Design review of the part built by this model. Coordinates are the model's own, in mm. Face numbers are marked on the shaded views. A direction names the side the tool comes from. Round coordinates to 2 decimals unless told otherwise and drop trailing zeros. Loops run counter-clockwise (first coordinate to the right, second up) from the corner with the lowest first, then second, coordinate; pieces in that order, holes last. Notation, with made-up numbers: (37, 70) - (50, 70) arc R23 ccw to (50, 93) - close; hole circle Ø11 at (-23, 10). An arc over 180 degrees is marked (long way). Return JSON: item names as keys, results as strings. Group by question number.
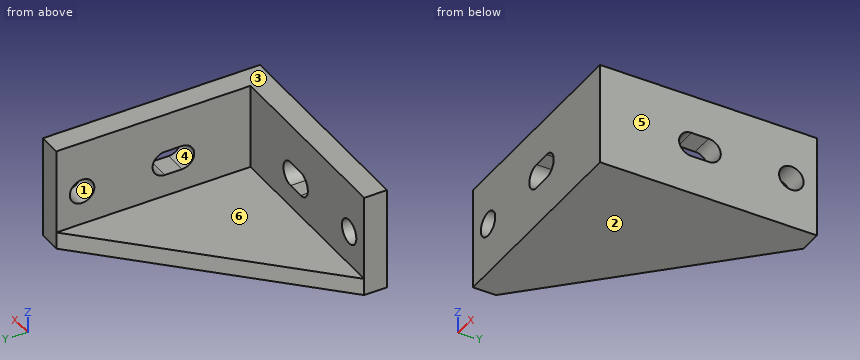
from build123d import *

# Parameters (mm, degrees)
EXTRUDE_1_DEPTH     = 9
EXTRUDE_2_DEPTH     = 3
SKETCH_4_R          = 2.15
CUT_EXTRUDE_1_DEPTH = 52.778373864


with BuildPart() as part:
    # 草图1 → 凸台-拉伸1 (new, symmetric)
    with BuildSketch(Plane.XY):
        Polygon((-38, 0), (0, 0), (0, 38), (-4, 38), (-4, 4), (-38, 4), align=None)
    extrude(amount=EXTRUDE_1_DEPTH, both=True)

    # 草图3 → 凸台-拉伸2 (add)
    with BuildSketch(Plane(origin=(0, 0, -9), x_dir=(-1, 0, 0), z_dir=(0, 0, -1))):
        Polygon((38, 4), (4, 38), (4, 4), align=None)
    extrude(amount=-EXTRUDE_2_DEPTH)

    # 草图4 → 切除-拉伸1 (cut, through all)
    with BuildSketch(Plane(origin=(0, 4, 0), x_dir=(1, 0, 0), z_dir=(0, 1, 0))):
        with Locations(Location((-33.5, 0, 0), (0, 0, 270))):
            Circle(SKETCH_4_R)
        with BuildLine():
            Line((-16, -2.15), (-19, -2.15))
            ThreePointArc((-19, -2.15), (-21.15, 0), (-19, 2.15))
            Line((-19, 2.15), (-16, 2.15))
            ThreePointArc((-16, 2.15), (-13.85, 0), (-16, -2.15))
        make_face()
    cut_extrude_1 = extrude(amount=-CUT_EXTRUDE_1_DEPTH, mode=Mode.SUBTRACT)

    # 镜向1: 切除-拉伸1 across plane
    add(cut_extrude_1.mirror(Plane(origin=(0, 0, 0), x_dir=(0, 0, 1), z_dir=(-0.7071067811865477, -0.7071067811865475, 0))), mode=Mode.SUBTRACT)


solid = part.part
Q1. Add section A-A, the plane z = 0. State the section outline as (x, y) points, plus the area to 3 significant figures.
Q2. For line 1 (X direction, y = 0.8, z = 0); line 2 (Y direction, x = -2.45, z = 0); line 3 (Z direction, x = -18, y = 3), list the stretches that pass through material, from the lowest coordinate up.
Q3. Draft analysis for pull direction Z (two halves, no side actions). For the marked faces 1, 2 and 3, state which applies: pulls with the +Z half, pulls with the -Z half, needs draft (parallel to the pull), parting line crosses it, or undercut.
Q4. Insertion check: pin 1 Ø1 at (x, z) = (-20.5, 5) entering from +Y; pin 2 Ø10 at (y, z) = (24, 7) entering from -X; pin 3 Ø17 at (x, y) = (-18.5, 13) entering from +Z. Each pin has a flat end and moves straight along its axis. Give the tip position at first contact, or say it passes through.
Q5. Add section D-D, the plane x = -8. State the section outline as (y, z) points.
Q6. Add section B-B, the plane y = 33.5. State the section outline as (x, z) points, plus the area to 3 significant figures.
Q7. Add section C-C, the plane x = -20.5. State the section outline as (y, z) points, plus the area to 3 significant figures.
Q8. Tool access review of the marked faces 4, 5 and 6: name each direction out of +Z, -Z, +X, -X, +Y, -Y from which nothing blocks a thin tool from reaching the whole face with its end or side.
Evaluation:
{
 "1": {"outline": "(-38, 0) - (-35.65, 0) - (-35.65, 4) - (-38, 4) - close; (-31.35, 0) - (-21.15, 0) - (-21.15, 4) - (-31.35, 4) - close; (-13.85, 0) - (0, 0) - (0, 13.85) - (-4, 13.85) - (-4, 4) - (-13.85, 4) - close; (-4, 21.15) - (0, 21.15) - (0, 31.35) - (-4, 31.35) - close; (-4, 35.65) - (0, 35.65) - (0, 38) - (-4, 38) - close", "area": "195 mm²"},
 "2": {"line 1": "-38 to -35.65, -31.35 to -21.15, -13.85 to 0", "line 2": "0 to 13.85, 21.15 to 31.35, 35.65 to 38", "line 3": "-9 to -2.15, 2.15 to 9"},
 "3": {"face 1": "undercut", "face 2": "pulls with the -Z half", "face 3": "pulls with the +Z half"},
 "4": {"pin 1": "y = 4", "pin 2": "x = -4", "pin 3": "z = -6"},
 "5": {"outline": "(0, -9) - (34, -9) - (34, -6) - (4, -6) - (4, 9) - (0, 9) - close"},
 "6": {"outline": "(-8.5, -9) - (0, -9) - (0, -2.15) - (-4, -2.15) - (-4, -6) - (-8.5, -6) - close; (-4, 2.15) - (0, 2.15) - (0, 9) - (-4, 9) - close", "area": "68.3 mm²"},
 "7": {"outline": "(0, -9) - (21.5, -9) - (21.5, -6) - (4, -6) - (4, -1.54) - (0, -1.54) - close; (0, 1.54) - (4, 1.54) - (4, 9) - (0, 9) - close", "area": "112 mm²"},
 "8": {"face 4": "+X, -X", "face 5": "+Z, -Z, +X, +Y, -Y", "face 6": "+Z, -X, +Y"}
}
